```python
from build123d import *

# Parameters (mm, degrees)
SKETCH1_W           = 95
SKETCH1_H           = 64
BOSS_EXTRUDE1_DEPTH = 2
SKETCH2_R           = 3.5
BOSS_EXTRUDE2_DEPTH = 2
FILLET1_R           = 4
FILLET2_R           = 3
SKETCH3_R           = 1.5
CUT_EXTRUDE1_DEPTH  = 62.090097397
SKETCH4_W           = 75.8
SKETCH4_H           = 50.8
CUT_EXTRUDE2_DEPTH  = 62.090097397
CHAMFER1_SIZE       = 3
CHAMFER1_SIZE_2     = 2.100622615
FILLET3_R           = 5


with BuildPart() as part:
    # Sketch1 → Boss-Extrude1 (new body)
    with BuildSketch(Plane(origin=(0, 0, 0), x_dir=(1, 0, 0), z_dir=(0, 1, 0))):
        Rectangle(SKETCH1_W, SKETCH1_H)
    extrude(amount=BOSS_EXTRUDE1_DEPTH)

    # Sketch2 → Boss-Extrude2 (add)
    with BuildSketch(Plane(origin=(0, 2, 0), x_dir=(1, 0, 0), z_dir=(0, 1, 0))):
        with Locations((-48.5, -26)):
            Circle(SKETCH2_R)
        with Locations((-48.5, 26)):
            Circle(SKETCH2_R)
        with Locations((48.5, -26)):
            Circle(SKETCH2_R)
        with Locations((48.5, 26)):
            Circle(SKETCH2_R)
    extrude(amount=-BOSS_EXTRUDE2_DEPTH)

    # Fillet1
    # the kernel refuses this fillet: 4 mm, written as the material it adds along each edge
    with BuildSketch(Plane(origin=(-47.5, 0, -29.354101966), x_dir=(0, 0, -1), z_dir=(0, 1, 0))) as fillet1_piece_1:
        with BuildLine():
            CenterArc((3.565539249, 3.892847292), FILLET1_R, 202.68800958, 54.020199403)
            Line((-0.124936066, 2.349995403), (-0.198745572, 2.319138365))
            ThreePointArc((-0.198745572, 2.319138365), (0.061075022, 1.181565792), (-0.076665188, 0.022857143))
            Line((-0.076665188, 0.022857143), (0, -0.08))
            ThreePointArc((0, -0.08), (1.322949017, -0.08), (2.627505209, -0.077856946))
            Line((2.627505209, -0.077856946), (2.645898034, 0))
        make_face()
    extrude(amount=2)
    with BuildSketch(Plane(origin=(-47.5, 0, -22.645898034), x_dir=(-0.998147228603926, 0, -0.06084496717315217), z_dir=(0, 1, 0)), Plane(origin=(47.5, 0, 22.645898034), x_dir=(0.9981472286039255, 0, 0.06084496717316137), z_dir=(0, 1, 0))) as fillet1_piece_2:
        with BuildLine():
            CenterArc((3.778429137, 3.756620131), FILLET1_R, 183.48831444, 66.421821522)
            Line((-0.214159778, 3.513240263), (-0.294011556, 3.508372665))
            Line((-0.294011556, 3.508372665), (-0.079851778, -0.004867597))
            Line((-0.079851778, -0.004867597), (0.027479485, -0.075132403))
            ThreePointArc((0.027479485, -0.075132403), (1.202227453, 0.132957385), (2.376975421, -0.075132403))
            Line((2.376975421, -0.075132403), (2.404454905, 0))
        make_face()
    extrude(amount=2)
    with BuildSketch(Plane(origin=(-47.5, 0, 22.645898034), x_dir=(0, 0, -1), z_dir=(0, 1, 0)), Plane(origin=(47.5, 0, -22.645898034), x_dir=(0, 0, 1), z_dir=(0, 1, 0))) as fillet1_piece_3:
        with BuildLine():
            CenterArc((3.519761576, 4), FILLET1_R, 203.578178478, 66.421821522)
            Line((-0.14629898, 2.4), (-0.219620191, 2.368))
            ThreePointArc((-0.219620191, 2.368), (0.059561556, 1.208089788), (-0.076665188, 0.022857143))
            Line((-0.076665188, 0.022857143), (0, -0.08))
            Line((0, -0.08), (3.519761576, -0.08))
            Line((3.519761576, -0.08), (3.519761576, 0))
        make_face()
    extrude(amount=2)
    with BuildSketch(Plane(origin=(-47.5, 0, 29.354101966), x_dir=(-0.9985897627331907, 0, -0.05308941292263453), z_dir=(0, 1, 0)), Plane(origin=(47.5, 0, -29.354101966), x_dir=(0.9985897627331903, 0, 0.053089412922639356), z_dir=(0, 1, 0))) as fillet1_piece_4:
        with BuildLine():
            CenterArc((3.698065068, 3.76717997), FILLET1_R, 196.335021008, 54.020199403)
            Line((-0.140469173, 2.64216669), (-0.217239858, 2.619666424))
            ThreePointArc((-0.217239858, 2.619666424), (-0.150121768, 1.316836192), (-0.079887181, -0.004247153))
            Line((-0.079887181, -0.004247153), (0.026895019, -0.075343599))
            ThreePointArc((0.026895019, -0.075343599), (1.176657067, 0.123717526), (2.326419115, -0.075343599))
            Line((2.326419115, -0.075343599), (2.353314134, 0))
        make_face()
    extrude(amount=2)
    with BuildSketch(Plane(origin=(47.5, 0, 29.354101966), x_dir=(0.9985897627331901, 0, -0.05308941292264221), z_dir=(0, 1, 0))) as fillet1_piece_5:
        with BuildLine():
            CenterArc((3.698065068, -3.76717997), FILLET1_R, 109.64477959, 54.020199403)
            Line((-0.140469173, -2.64216669), (-0.217239858, -2.619666424))
            ThreePointArc((-0.217239858, -2.619666424), (-0.150121768, -1.316836192), (-0.079887181, 0.004247153))
            Line((-0.079887181, 0.004247153), (0.026895019, 0.075343599))
            ThreePointArc((0.026895019, 0.075343599), (1.176657067, -0.123717526), (2.326419115, 0.075343599))
            Line((2.326419115, 0.075343599), (2.353314134, 0))
        make_face()
    extrude(amount=2)

    # Fillet2
    fillet2_edges = [part.edges().sort_by_distance(p)[0] for p in [
        (-47.5, 1, -32),
        (47.5, 1, -32),
        (47.5, 1, 32),
        (-47.5, 1, 32),
    ]]
    fillet(fillet2_edges, radius=FILLET2_R)

    # Sketch3 → Cut-Extrude1 (cut, through all)
    with BuildSketch(Plane(origin=(0, 2, 0), x_dir=(1, 0, 0), z_dir=(0, 1, 0))):
        with Locations(Location((48.5, -26, 0), (0, 0, 270))):
            Circle(SKETCH3_R)
        with Locations(Location((48.5, 26, 0), (0, 0, 270))):
            Circle(SKETCH3_R)
        with Locations(Location((-48.5, 26, 0), (0, 0, 270))):
            Circle(SKETCH3_R)
        with Locations(Location((-48.5, -26, 0), (0, 0, 270))):
            Circle(SKETCH3_R)
    extrude(amount=-CUT_EXTRUDE1_DEPTH, mode=Mode.SUBTRACT)

    # Sketch4 → Cut-Extrude2 (cut, through all)
    with BuildSketch(Plane(origin=(0, 2, 0), x_dir=(1, 0, 0), z_dir=(0, 1, 0))):
        with Locations((3.429138832, 1.001657313)):
            Rectangle(SKETCH4_W, SKETCH4_H)
    extrude(amount=-CUT_EXTRUDE2_DEPTH, mode=Mode.SUBTRACT)

    # Chamfer1
    # the kernel refuses this chamfer: 3, 2.100622615 mm, written as the material it takes off along each edge
    with BuildSketch(Plane(origin=(-34.470861168, 2, -26.401657313), x_dir=(-0.9997533347641299, 0.022209674198456996, 0), z_dir=(0, 0, 1)), Plane(origin=(41.329138832, 2, 24.398342687), x_dir=(0.9997533347641299, 0.022209674198456996, 0), z_dir=(0, 0, -1))) as chamfer1_piece_1:
        Polygon((CHAMFER1_SIZE * 0.999753334764, CHAMFER1_SIZE * 0.0222096741985), (-CHAMFER1_SIZE_2 * 0.0222096741945, CHAMFER1_SIZE_2 * 0.999753334588), (0, 0), align=None)
    extrude(amount=50.8, mode=Mode.SUBTRACT)
    with BuildSketch(Plane(origin=(-34.470861168, 2, 24.398342687), x_dir=(0, 0.022209674198456996, 0.9997533347641299), z_dir=(1, 0, 0)), Plane(origin=(41.329138832, 2, -26.401657313), x_dir=(0, 0.022209674198456972, -0.99975333476413), z_dir=(-1, 0, 0))) as chamfer1_piece_2:
        Polygon((CHAMFER1_SIZE * 0.999753334764, CHAMFER1_SIZE * 0.0222096741985), (-CHAMFER1_SIZE_2 * 0.0222096741945, CHAMFER1_SIZE_2 * 0.999753334588), (0, 0), align=None)
    extrude(amount=75.8, mode=Mode.SUBTRACT)
    with BuildSketch(Plane(origin=(-34.470861168, 2, -34.149314004), x_dir=(-0.9997533347641299, 0.022209674198456996, 0), z_dir=(0, 0, 1))) as chamfer1_piece_3a_section:
        Polygon((CHAMFER1_SIZE * 0.999753334764, CHAMFER1_SIZE * 0.0222096741985), (-CHAMFER1_SIZE_2 * 0.0222096741945, CHAMFER1_SIZE_2 * 0.999753334588), (0, 0), align=None)
    chamfer1_piece_3a = extrude(amount=58.547656691, mode=Mode.PRIVATE)
    chamfer1_piece_3a = split(chamfer1_piece_3a, bisect_by=Plane(origin=(-35.470351342, 1.318269678, -26.401657313), z_dir=(0, 0, -1)), keep=Keep.TOP, mode=Mode.PRIVATE)
    with BuildSketch(Plane(origin=(41.329138832, 2, -26.401657313), x_dir=(0, 0.022209674198456972, -0.99975333476413), z_dir=(-1, 0, 0))) as chamfer1_piece_3b_section:
        Polygon((CHAMFER1_SIZE * 0.999753334764, CHAMFER1_SIZE * 0.0222096741985), (-CHAMFER1_SIZE_2 * 0.0222096741945, CHAMFER1_SIZE_2 * 0.999753334588), (0, 0), align=None)
    chamfer1_piece_3b = extrude(amount=83.547656691, mode=Mode.PRIVATE)
    chamfer1_piece_3b = split(chamfer1_piece_3b, bisect_by=Plane(origin=(-34.470861168, 1.318269678, -27.401147488), z_dir=(-1, 0, 0)), keep=Keep.TOP, mode=Mode.PRIVATE)
    chamfer1_piece_3 = chamfer1_piece_3a & chamfer1_piece_3b
    add(chamfer1_piece_3, mode=Mode.SUBTRACT)
    with BuildSketch(Plane(origin=(-34.470861168, 2, -26.401657313), x_dir=(-0.9997533347641299, 0.022209674198456996, 0), z_dir=(0, 0, 1))) as chamfer1_piece_4a_section:
        Polygon((CHAMFER1_SIZE * 0.999753334764, CHAMFER1_SIZE * 0.0222096741985), (-CHAMFER1_SIZE_2 * 0.0222096741945, CHAMFER1_SIZE_2 * 0.999753334588), (0, 0), align=None)
    chamfer1_piece_4a = extrude(amount=58.547656691, mode=Mode.PRIVATE)
    chamfer1_piece_4a = split(chamfer1_piece_4a, bisect_by=Plane(origin=(-35.470351342, 1.318269678, 24.398342687), z_dir=(0, 0, 1)), keep=Keep.TOP, mode=Mode.PRIVATE)
    with BuildSketch(Plane(origin=(-42.218517859, 2, 24.398342687), x_dir=(0, 0.022209674198456996, 0.9997533347641299), z_dir=(1, 0, 0))) as chamfer1_piece_4b_section:
        Polygon((CHAMFER1_SIZE * 0.999753334764, CHAMFER1_SIZE * 0.0222096741985), (-CHAMFER1_SIZE_2 * 0.0222096741945, CHAMFER1_SIZE_2 * 0.999753334588), (0, 0), align=None)
    chamfer1_piece_4b = extrude(amount=83.547656691, mode=Mode.PRIVATE)
    chamfer1_piece_4b = split(chamfer1_piece_4b, bisect_by=Plane(origin=(-34.470861168, 1.318269678, 25.397832861), z_dir=(-1, 0, 0)), keep=Keep.TOP, mode=Mode.PRIVATE)
    chamfer1_piece_4 = chamfer1_piece_4a & chamfer1_piece_4b
    add(chamfer1_piece_4, mode=Mode.SUBTRACT)
    with BuildSketch(Plane(origin=(41.329138832, 2, 32.145999377), x_dir=(0.9997533347641299, 0.022209674198456996, 0), z_dir=(0, 0, -1))) as chamfer1_piece_5a_section:
        Polygon((CHAMFER1_SIZE * 0.999753334764, CHAMFER1_SIZE * 0.0222096741985), (-CHAMFER1_SIZE_2 * 0.0222096741945, CHAMFER1_SIZE_2 * 0.999753334588), (0, 0), align=None)
    chamfer1_piece_5a = extrude(amount=58.547656691, mode=Mode.PRIVATE)
    chamfer1_piece_5a = split(chamfer1_piece_5a, bisect_by=Plane(origin=(42.328629006, 1.318269678, 24.398342687), z_dir=(0, 0, 1)), keep=Keep.TOP, mode=Mode.PRIVATE)
    with BuildSketch(Plane(origin=(-34.470861168, 2, 24.398342687), x_dir=(0, 0.022209674198456996, 0.9997533347641299), z_dir=(1, 0, 0))) as chamfer1_piece_5b_section:
        Polygon((CHAMFER1_SIZE * 0.999753334764, CHAMFER1_SIZE * 0.0222096741985), (-CHAMFER1_SIZE_2 * 0.0222096741945, CHAMFER1_SIZE_2 * 0.999753334588), (0, 0), align=None)
    chamfer1_piece_5b = extrude(amount=83.547656691, mode=Mode.PRIVATE)
    chamfer1_piece_5b = split(chamfer1_piece_5b, bisect_by=Plane(origin=(41.329138832, 1.318269678, 25.397832861), z_dir=(1, 0, 0)), keep=Keep.TOP, mode=Mode.PRIVATE)
    chamfer1_piece_5 = chamfer1_piece_5a & chamfer1_piece_5b
    add(chamfer1_piece_5, mode=Mode.SUBTRACT)
    with BuildSketch(Plane(origin=(49.076795523, 2, -26.401657313), x_dir=(0, 0.022209674198456944, -0.9997533347641299), z_dir=(-1, 0, 0))) as chamfer1_piece_6a_section:
        Polygon((CHAMFER1_SIZE * 0.999753334764, CHAMFER1_SIZE * 0.0222096741985), (-CHAMFER1_SIZE_2 * 0.0222096741945, CHAMFER1_SIZE_2 * 0.999753334588), (0, 0), align=None)
    chamfer1_piece_6a = extrude(amount=83.547656691, mode=Mode.PRIVATE)
    chamfer1_piece_6a = split(chamfer1_piece_6a, bisect_by=Plane(origin=(41.329138832, 1.318269678, -27.401147488), z_dir=(1, 0, 0)), keep=Keep.TOP, mode=Mode.PRIVATE)
    with BuildSketch(Plane(origin=(41.329138832, 2, 24.398342687), x_dir=(0.9997533347641299, 0.022209674198456996, 0), z_dir=(0, 0, -1))) as chamfer1_piece_6b_section:
        Polygon((CHAMFER1_SIZE * 0.999753334764, CHAMFER1_SIZE * 0.0222096741985), (-CHAMFER1_SIZE_2 * 0.0222096741945, CHAMFER1_SIZE_2 * 0.999753334588), (0, 0), align=None)
    chamfer1_piece_6b = extrude(amount=58.547656691, mode=Mode.PRIVATE)
    chamfer1_piece_6b = split(chamfer1_piece_6b, bisect_by=Plane(origin=(42.328629006, 1.318269678, -26.401657313), z_dir=(0, 0, -1)), keep=Keep.TOP, mode=Mode.PRIVATE)
    chamfer1_piece_6 = chamfer1_piece_6a & chamfer1_piece_6b
    add(chamfer1_piece_6, mode=Mode.SUBTRACT)

    # Fillet3
    fillet3_edges = [part.edges().sort_by_distance(p)[0] for p in [
        (3.429138832, 2, 27.398342687),
        (44.329138832, 2, -1.001657313),
        (3.429138832, 2, -29.401657313),
        (-37.470861168, 2, -1.001657313),
    ]]
    fillet(fillet3_edges, radius=FILLET3_R)


solid = part.part
```
Model file for the job. Use its own axes, mm. A direction names the side the tool comes from. Coordinates: 2 decimals unless noted, no trailing zeros. Loops run counter-clockwise (first coordinate to the right, second up) from the corner with the lowest first, then second, coordinate; pieces in that order, holes last. Notation, with made-up numbers: M 28,-11.5 L 75,-11.5 A21 ccw 75,4.5 Z; hole C 58.5,-19 d1. An arc over 180 degrees is marked long. Use CSV: the item, a comma, the result in double quotes. Start each with the question number.
1. Band-saw the part on C-C, the plane y = 0.4. List the corners of the cut face in (x, z).
2. Flat gauge pins, fed straight in: pin 1 (1 mm diameter, centred on y = 1.5, z = 22.5, fed in from +X); pin 2 (1 mm diameter, centred on y = 1, z = 8, fed in from +X); pin 3 (10 mm diameter, centred on x = -30.5, z = 15.5, fed in from +Y). Where does each tip first touch, or does it go through?
3. Two-plate mould, pull along Z, no slides. Class faces 1 (the flat face through (-6, 0, 26)), 2 (the cylindrical face through (2.834, 1.775, 27.492)), 3 (the cylindrical face through (-46.98, 1.01, 31.66)): pulls with the +Z half, pulls with the -Z half, needs draft (parallel to the pull), parting line crosses it, or undercut.
4. Probe probe 1 along X at (y, z) = (0.6, 25); probe 2 along X at (y, z) = (1.5, 26); probe 3 along X at (y, z) = (0.9, -17.5). List the from-to ranges inside material, lowest first. Write a range as [from, to].
5. Band-saw the part on A-A, the plane z = 16. List the corners of the cut face in (x, y).
6. Tool access for faces 4 (the cylindrical face through (47.02, 1.01, -31.64)), 5 (the flat face through (-47.5, 1, 0)), 6 (the flat face through (47.5, 1, 0)): list every direction of +Z, -Z, +X, -X, +Y, -Y with a clear straight run to the whole face (end or side of a thin tool).
7. Band-saw the part on B-B, the plane x = 38. List the corners of the cut face in (y, z).
Entries:
1,outline,"M -49.9,-22.79 A3.5 ccw -49.85,-29.23 A4 cw -48.08,-30.68 A3 ccw -45.59,-32 L 45.59,-32 A3 ccw 48.08,-30.68 A4 cw 49.85,-29.23 A3.5 ccw 49.9,-22.79 A4 cw 47.5,-19.13 L 47.5,19.13 A4 cw 49.9,22.79 A3.5 ccw 49.85,29.23 A4 cw 48.08,30.68 A3 ccw 45.59,32 L -45.59,32 A3 ccw -48.08,30.68 A4 cw -49.85,29.23 A3.5 ccw -49.9,22.79 A4 cw -47.5,19.13 L -47.5,-19.13 A4 cw Z; hole C -48.5,-26 d3; hole C -48.5,26 d3; hole M -35.19,-27.12 L 42.04,-27.12 L 42.04,25.11 L -35.19,25.11 Z; hole C 48.5,-26 d3; hole C 48.5,26 d3"
2,pin 1,"stops at x = 50.3"
2,pin 2,"stops at x = 47.5"
2,pin 3,"stops at y = 0.62"
3,face 1,"needs draft"
3,face 2,"undercut"
3,face 3,"pulls with the +Z half"
4,probe 1,"x = [-51.85, -49.62], [-47.38, -35.47], [42.33, 47.38], [49.62, 51.85]"
4,probe 2,"x = [-52, -50], [-47, -36.87], [43.73, 47], [50, 52]"
4,probe 3,"x = [-47.5, -35.9], [42.76, 47.5]"
5,outline,"M -47.5,0 L -34.61,0 L -36.18,1.1 A5 ccw -39.05,2 L -47.5,2 Z; M 41.47,0 L 47.5,0 L 47.5,2 L 45.91,2 A5 ccw 43.04,1.1 Z"
6,face 4,"-Z, +X, +Y, -Y"
6,face 5,"-X, +Y, -Y"
6,face 6,"+X, +Y, -Y"
7,outline,"M 0,-32 L 2,-32 L 2,-30.98 A5 ccw 1.1,-28.11 L 0,-26.55 Z; M 0,24.54 L 1.1,26.11 A5 ccw 2,28.97 L 2,32 L 0,32 Z"
